Could you check a few things on this model? Use its own coordinates, in mm. A direction names the side the tool comes from. Round coordinates to 2 decimals unless told otherwise and drop trailing zeros. Write each loop counter-clockwise with the first axis right and the second up, starting at its lowest first coordinate (ties: lowest second). Pieces come first, ordered by that corner, then holes. Notation, with made-up numbers: (-34.75, 32) -> (0.25, 32) arc R21 cw to (0.25, 47) -> close; hole circle Ø4 at (-25, 1.5). An arc over 180 degrees is marked (long way). Answer in a Markdown table with one row per item.
from build123d import *

# Parameters (mm, degrees)
BOSS_EXTRUDE1_DEPTH = 1
CUT_EXTRUDE1_REACH  = 3
SKETCH2_R           = 1.75


with BuildPart() as part:
    # Sketch1 → Boss-Extrude1 (new body)
    with BuildSketch(Plane(origin=(0, 0, 0), x_dir=(1, 0, 0), z_dir=(0, 1, 0))):
        with BuildLine():
            Line((39.4, -105), (39.4, 0))
            Line((39.4, 0), (40, 0))
            Line((40, 0), (40, -105))
            ThreePointArc((40, -105), (41.464466094, -108.535533906), (45, -110))
            Line((45, -110), (54.4, -110))
            ThreePointArc((54.4, -110), (57.935533906, -108.535533906), (59.4, -105))
            Line((59.4, -105), (59.4, 0))
            Line((59.4, 0), (60, 0))
            Line((60, 0), (60, -105))
            ThreePointArc((60, -105), (61.464466094, -108.535533906), (65, -110))
            Line((65, -110), (74.4, -110))
            ThreePointArc((74.4, -110), (77.935533906, -108.535533906), (79.4, -105))
            Line((79.4, -105), (79.4, 0))
            Line((79.4, 0), (80, 0))
            Line((80, 0), (80, -105))
            ThreePointArc((80, -105), (81.464466094, -108.535533906), (85, -110))
            Line((85, -110), (94.4, -110))
            ThreePointArc((94.4, -110), (97.935533906, -108.535533906), (99.4, -105))
            Line((99.4, -105), (99.4, 0))
            Line((99.4, 0), (100, 0))
            Line((100, 0), (100, -105))
            ThreePointArc((100, -105), (101.464466094, -108.535533906), (105, -110))
            Line((105, -110), (114.4, -110))
            ThreePointArc((114.4, -110), (117.935533906, -108.535533906), (119.4, -105))
            Line((119.4, -105), (119.4, 0))
            Line((119.4, 0), (120, 0))
            Line((120, 0), (120, -105))
            ThreePointArc((120, -105), (121.464466094, -108.535533906), (125, -110))
            Line((125, -110), (134.4, -110))
            ThreePointArc((134.4, -110), (137.935533906, -108.535533906), (139.4, -105))
            Line((139.4, -105), (139.4, 0))
            Line((139.4, 0), (140, 0))
            Line((140, 0), (140, 20))
            Line((140, 20), (5, 20))
            ThreePointArc((5, 20), (1.464466094, 18.535533906), (0, 15))
            Line((0, 15), (0, -105))
            ThreePointArc((0, -105), (1.464466094, -108.535533906), (5, -110))
            Line((5, -110), (14.4, -110))
            ThreePointArc((14.4, -110), (17.935533906, -108.535533906), (19.4, -105))
            Line((19.4, -105), (19.4, 0))
            Line((19.4, 0), (20, 0))
            Line((20, 0), (20, -105))
            ThreePointArc((20, -105), (21.464466094, -108.535533906), (25, -110))
            Line((25, -110), (34.4, -110))
            ThreePointArc((34.4, -110), (37.935533906, -108.535533906), (39.4, -105))
        make_face()
    extrude(amount=BOSS_EXTRUDE1_DEPTH)

    # Sketch2 → Cut-Extrude1 (cut, up to next)
    with BuildSketch(Plane(origin=(0, 1, 0), x_dir=(1, 0, 0), z_dir=(0, 1, 0)), mode=Mode.PRIVATE) as cut_extrude1_sk1:
        with Locations((10, 10)):
            Circle(SKETCH2_R)
    cut_extrude1_tool1 = extrude(cut_extrude1_sk1.sketch, amount=-CUT_EXTRUDE1_REACH, mode=Mode.PRIVATE) & part.part
    add(cut_extrude1_tool1.solids().sort_by_distance((10, 1, -10))[0], mode=Mode.SUBTRACT)
    # Sketch2 → Cut-Extrude1 (cut, up to next)
    with BuildSketch(Plane(origin=(0, 1, 0), x_dir=(1, 0, 0), z_dir=(0, 1, 0)), mode=Mode.PRIVATE) as cut_extrude1_sk2:
        with Locations((40, 10)):
            Circle(SKETCH2_R)
    cut_extrude1_tool2 = extrude(cut_extrude1_sk2.sketch, amount=-CUT_EXTRUDE1_REACH, mode=Mode.PRIVATE) & part.part
    add(cut_extrude1_tool2.solids().sort_by_distance((40, 1, -10))[0], mode=Mode.SUBTRACT)
    # Sketch2 → Cut-Extrude1 (cut, up to next)
    with BuildSketch(Plane(origin=(0, 1, 0), x_dir=(1, 0, 0), z_dir=(0, 1, 0)), mode=Mode.PRIVATE) as cut_extrude1_sk3:
        with Locations((70, 10)):
            Circle(SKETCH2_R)
    cut_extrude1_tool3 = extrude(cut_extrude1_sk3.sketch, amount=-CUT_EXTRUDE1_REACH, mode=Mode.PRIVATE) & part.part
    add(cut_extrude1_tool3.solids().sort_by_distance((70, 1, -10))[0], mode=Mode.SUBTRACT)
    # Sketch2 → Cut-Extrude1 (cut, up to next)
    with BuildSketch(Plane(origin=(0, 1, 0), x_dir=(1, 0, 0), z_dir=(0, 1, 0)), mode=Mode.PRIVATE) as cut_extrude1_sk4:
        with Locations((100, 10)):
            Circle(SKETCH2_R)
    cut_extrude1_tool4 = extrude(cut_extrude1_sk4.sketch, amount=-CUT_EXTRUDE1_REACH, mode=Mode.PRIVATE) & part.part
    add(cut_extrude1_tool4.solids().sort_by_distance((100, 1, -10))[0], mode=Mode.SUBTRACT)
    # Sketch2 → Cut-Extrude1 (cut, up to next)
    with BuildSketch(Plane(origin=(0, 1, 0), x_dir=(1, 0, 0), z_dir=(0, 1, 0)), mode=Mode.PRIVATE) as cut_extrude1_sk5:
        with Locations((130, 10)):
            Circle(SKETCH2_R)
    cut_extrude1_tool5 = extrude(cut_extrude1_sk5.sketch, amount=-CUT_EXTRUDE1_REACH, mode=Mode.PRIVATE) & part.part
    add(cut_extrude1_tool5.solids().sort_by_distance((130, 1, -10))[0], mode=Mode.SUBTRACT)


solid = part.part
1) Thinking about a two-plate mould opening in Z: for faces 1 (the face through (131.669, 0.507, -10.526)), 2 (the face through (57.9, 0.49, 108.57)), 3 (the face through (69, 1, 44)), 4 (the face through (10.9, 0.5, -11.5)), which applies, +Z half, -Z half, draft (parallel to the pull), parting line (faces both ways), or undercut?
Findings:
| item | result |
|---|---|
| face 1 | undercut |
| face 2 | +Z half |
| face 3 | draft |
| face 4 | undercut |
2) Imagine slicing it at C-C, the plane z = 42.5. Please give me the cut outline in (x, y), plus the area to 3 significant figures.
Findings:
| item | result |
|---|---|
| outline | (0, 0) -> (19.4, 0) -> (19.4, 1) -> (0, 1) -> close; (20, 0) -> (39.4, 0) -> (39.4, 1) -> (20, 1) -> close; (40, 0) -> (59.4, 0) -> (59.4, 1) -> (40, 1) -> close; (60, 0) -> (79.4, 0) -> (79.4, 1) -> (60, 1) -> close; (80, 0) -> (99.4, 0) -> (99.4, 1) -> (80, 1) -> close; (100, 0) -> (119.4, 0) -> (119.4, 1) -> (100, 1) -> close; (120, 0) -> (139.4, 0) -> (139.4, 1) -> (120, 1) -> close |
| area | 136 mm^2 |
3) Imagine slicing it at B-B, the plane x = 70. Please give me the cut outline in (y, z), plus the area to 4 significant figures.
Findings:
| item | result |
|---|---|
| outline | (0, -20) -> (1, -20) -> (1, -11.75) -> (0, -11.75) -> close; (0, -8.25) -> (1, -8.25) -> (1, 110) -> (0, 110) -> close |
| area | 126.5 mm^2 |
4) Imagine slicing it at D-D, the plane y = 0.8. Count the separate pieces of the cut face and the enclosed holes in it, plus the area to 3 significant figures.
Findings:
| item | result |
|---|---|
| separate pieces | 1 |
| enclosed holes | 5 |
| area | 17,600 mm^2 |
5) For faces 5 (the face through (1.43, 0.49, 108.5)), 6 (the face through (117.9, 0.49, 108.57)), which set-ups out of +Z, -Z, +X, -X, +Y, -Y let a thin tool reach every point of the face, with its end or its side?
Findings:
| item | result |
|---|---|
| face 5 | +Z, -X, +Y, -Y |
| face 6 | +Z, +Y, -Y |
6) Please list where these lines run through material, in increasing order: line 1 (X direction, y = 0.5, z = -10); line 2 (Z direction, x = 130, y = 0.3); line 3 (Z direction, x = 97, y = 0.6).
Findings:
| item | result |
|---|---|
| line 1 | x = 0 to 8.25, 11.75 to 38.25, 41.75 to 68.25, 71.75 to 98.25, 101.75 to 128.25, 131.75 to 140 |
| line 2 | z = -20 to -11.75, -8.25 to 110 |
| line 3 | z = -20 to 109.27 |
7) Imagine slicing it at A-A, the plane z = -10. Please give me the cut outline in (x, y), plus the area to 4 significant figures.
Findings:
| item | result |
|---|---|
| outline | (0, 0) -> (8.25, 0) -> (8.25, 1) -> (0, 1) -> close; (11.75, 0) -> (38.25, 0) -> (38.25, 1) -> (11.75, 1) -> close; (41.75, 0) -> (68.25, 0) -> (68.25, 1) -> (41.75, 1) -> close; (71.75, 0) -> (98.25, 0) -> (98.25, 1) -> (71.75, 1) -> close; (101.75, 0) -> (128.25, 0) -> (128.25, 1) -> (101.75, 1) -> close; (131.75, 0) -> (140, 0) -> (140, 1) -> (131.75, 1) -> close |
| area | 122.5 mm^2 |
8) For pin 1 (0.5 mm diameter, centred on y = 0.5, z = 57.5, fed in from +X), with a flat end and sliding along its axis, tell me the tip position at first contact or that it passes through.
Findings:
| item | result |
|---|---|
| pin 1 | stops at x = 139.4 |
